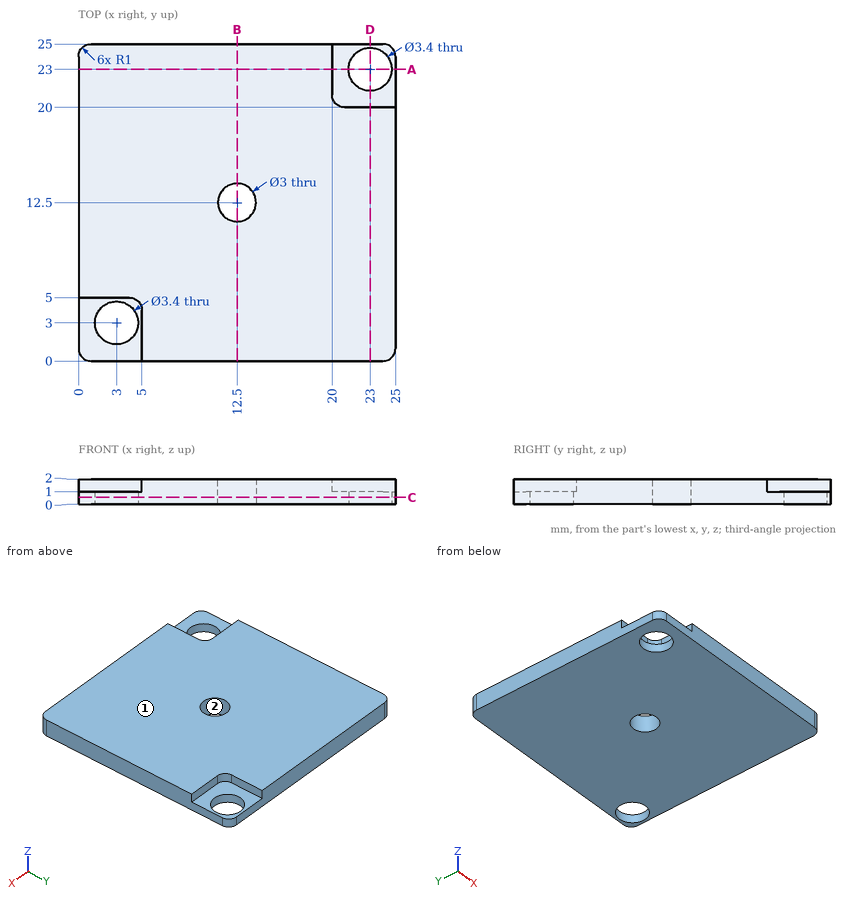
Here's the drawing with two shaded views (mm, measured from the low corner). I have some questions. Round coordinates to 2 decimals unless told otherwise and drop trailing zeros. Write each loop counter-clockwise with the first axis right and the second up, starting at its lowest first coordinate (ties: lowest second). Pieces come first, ordered by that corner, then holes. Notation, with made-up numbers: M -26,87.25 L -13,87.25 A19 ccw -13,124.25 Z; hole C -35.5,89 d8. An arc over 180 degrees is marked long. Answer in a Markdown table with one row per item. Add a question column.
Q1. Imagine slicing it at B-B (x = 12.5). Please give me the cut outline in (y, z).
Q2. Will these pins go through, and if not, where does the flat tip stop? pin 1 Ø4.5 at (x, y) = (23, 23) entering from +Z; pin 2 Ø1.1 at (x, z) = (1.5, 1.5) entering from -Y; pin 3 Ø0.8 at (y, z) = (24, 1.5) entering from +X; pin 4 Ø0.8 at (y, z) = (2, 1.5) entering from -X.
Q3. If I drill on line 1 (Y direction, x = 12.5, z = 1.15); line 2 (Y direction, x = 3, z = 0.65); line 3 (Y direction, x = 23.25, z = 1.2), over which ranges is the centre line in solid material (lowest first)? Write a range as from..to.
Q4. Imagine slicing it at A-A (y = 23). Please give me the cut outline in (x, z).
Q5. If we mould it in two halves opening along X, with no side actions, what happens to the marked faces 1 and 2? For each: +X half, -X half, draft (parallel to the pull), parting line (faces both ways), or undercut.
Q6. Imagine slicing it at C-C (z = 0.55). Please give me the cut outline in (x, y).
Values:
| question | item | result |
|---|---|---|
| 1 | outline | M 0,0 L 11,0 L 11,2 L 0,2 Z; M 14,0 L 25,0 L 25,2 L 14,2 Z |
| 2 | pin 1 | z = 1 |
| 2 | pin 2 | y = 0 |
| 2 | pin 3 | x = 20 |
| 2 | pin 4 | x = 5 |
| 3 | line 1 | 0..11, 14..25 |
| 3 | line 2 | 0..1.3, 4.7..25 |
| 3 | line 3 | 0..20 |
| 4 | outline | M 0,0 L 21.3,0 L 21.3,1 L 20,1 L 20,2 L 0,2 Z; M 24.7,0 L 25,0 L 25,1 L 24.7,1 Z |
| 5 | face 1 | draft |
| 5 | face 2 | undercut |
| 6 | outline | M 0,1 A1 ccw 1,0 L 24,0 A1 ccw 25,1 L 25,24 A1 ccw 24,25 L 1,25 A1 ccw 0,24 Z; hole C 3,3 d3.4; hole C 12.5,12.5 d3; hole C 23,23 d3.4 |
